Here's how the part is built. I have some questions about the finished solid (model axes, mm). Face numbers are marked on the shaded views. Give positions to 0.01 mm unless a question says otherwise; leave off trailing zeros. Write each loop counter-clockwise with the first axis right and the second up, starting at its lowest first coordinate (ties: lowest second). Pieces come first, ordered by that corner, then holes. Notation, with made-up numbers: (-12, 75) -> (15, 75) arc R23 cw to (15, 106) -> close; hole circle Ø5 at (-16.75, 15.25). An arc over 180 degrees is marked (long way). Answer as CSV lines item,"result". Start each with the question number.
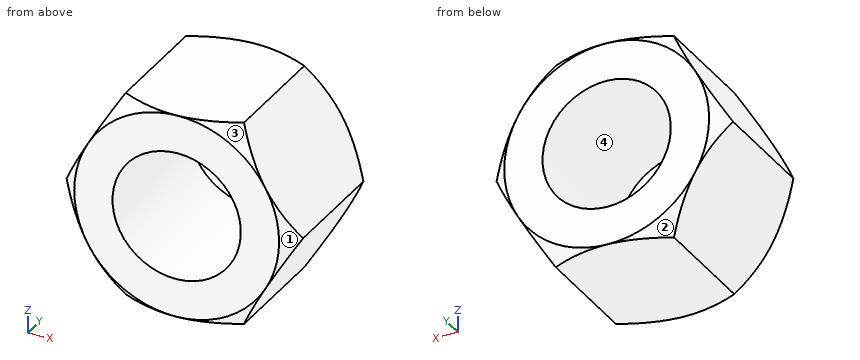
from build123d import *

# Parameters (mm, degrees)
BOSS_EXTRUDE1_DEPTH          = 30
CUT_EXTRUDE1_DEPTH           = 88.284496523
CUT_EXTRUDE1_DEPTH_BACK      = 88.284496523
SKETCH2_R                    = 26
SKETCH3_OUTSIDE_W            = 302.462
SKETCH3_OUTSIDE_H            = 289.622
SKETCH3_OUTSIDE_R            = 41.5
CUT_EXTRUDE2_DEPTH           = 88.284496523
CUT_EXTRUDE2_TAPER           = 45
CUT_EXTRUDE2_OTHER_WAY_DEPTH = 88.284496523


with BuildPart() as part:
    # Sketch1 → Boss-Extrude1 (new, symmetric)
    with BuildSketch(Plane(origin=(0, 0, 0), x_dir=(-1, 0, 0), z_dir=(0, 1, 0))):
        Polygon((47.920072343, 0), (23.960036171, 41.5), (-23.960036171, 41.5), (-47.920072343, 0), (-23.960036171, -41.5), (23.960036171, -41.5), align=None)
    extrude(amount=BOSS_EXTRUDE1_DEPTH, both=True)

    # Sketch2 → Cut-Extrude1 (cut, two sides: drawn at the far end of the back side and taken through both)
    with BuildSketch(Plane(origin=(0, 30, 0), x_dir=(-1, 0, 0), z_dir=(0, 1, 0)).offset(-CUT_EXTRUDE1_DEPTH_BACK)):
        with Locations(Location((0, 0, 0), (0, 0, 90))):
            Circle(SKETCH2_R)
    extrude(amount=CUT_EXTRUDE1_DEPTH + CUT_EXTRUDE1_DEPTH_BACK, mode=Mode.SUBTRACT)

    # Sketch3 outside → Cut-Extrude2 (cut)
    with BuildSketch(Plane(origin=(0, 30, 0), x_dir=(-1, 0, 0), z_dir=(0, 1, 0))):
        Rectangle(SKETCH3_OUTSIDE_W, SKETCH3_OUTSIDE_H)
        Circle(SKETCH3_OUTSIDE_R, mode=Mode.SUBTRACT)
    cut_extrude2 = extrude(amount=-CUT_EXTRUDE2_DEPTH, taper=CUT_EXTRUDE2_TAPER, mode=Mode.SUBTRACT)

    # Sketch3 outside → Cut-Extrude2 other way (cut)
    with BuildSketch(Plane(origin=(0, 30, 0), x_dir=(-1, 0, 0), z_dir=(0, 1, 0))):
        Rectangle(SKETCH3_OUTSIDE_W, SKETCH3_OUTSIDE_H)
        Circle(SKETCH3_OUTSIDE_R, mode=Mode.SUBTRACT)
    extrude(amount=CUT_EXTRUDE2_OTHER_WAY_DEPTH, mode=Mode.SUBTRACT)

    # Mirror1: Cut-Extrude2 across plane
    add(cut_extrude2.mirror(Plane.ZX), mode=Mode.SUBTRACT)


solid = part.part
Item 1: If I drill on line 1 (Z direction, x = 0, y = -5.5); line 2 (X direction, y = -12.5, z = 31); line 3 (X direction, y = 0.5, z = 6.5), over which ranges is the centre line in solid material (lowest first)? Write a range as [from, to].
Item 2: We'd pull the mould along Z, two halves only. Please class the marked faces 1, 2, 3 and 4: released by +Z, released by -Z, zero draft, split by the parting line, or undercut.
Item 3: If we section it at A-A (y = 7.5): Please give me the cut outline in (x, z), and give its area (3 significant figures).
Item 4: I'm going to push flat-ended pins straight in: pin 1 (2 mm diameter, centred on y = 1, z = -25.5, fed in from -X) (3 decimals); pin 2 (12 mm diameter, centred on y = 8.5, z = -23, fed in from +X); pin 3 (1 mm diameter, centred on y = -9.5, z = 22, fed in from +X). Where does each tip first touch, or does it pass through?
Final values:
1,line 1,"[-41.5, -26], [26, 41.5]"
1,line 2,"[-30.02, 30.02]"
1,line 3,"[-44.17, -25.17], [25.17, 44.17]"
2,face 1,"split by the parting line"
2,face 2,"released by -Z"
2,face 3,"released by +Z"
2,face 4,"undercut"
3,outline,"(-47.92, 0) -> (-23.96, -41.5) -> (23.96, -41.5) -> (47.92, 0) -> (23.96, 41.5) -> (-23.96, 41.5) -> close; hole circle Ø52 at (0, 0)"
3,area,"3,840 mm2"
4,pin 1,"x = -33.775"
4,pin 2,"x = 38.11"
4,pin 3,"x = 35.51"
